from build123d import *

# Parameters (mm, degrees)
F0_W      = 13.3
F0_H      = 8.82
F1_DEPTH  = 6.28
F2_R      = 3.95
F3_DEPTH  = 13.3
F4_W      = 8.82
F4_H      = 11.06
F5_DEPTH  = 3.54
F6_R      = 0.25
F7_W      = 4.685
F7_H      = 5.95
F9_R      = 3.25
F10_DEPTH = 9.4
F11_R     = 0.75
F12_DEPTH = 7.85
F13_R     = 0.875
F14_DEPTH = 1.5


with BuildPart() as f1:
    # F0 (on Top) → F1 (new body)
    with BuildSketch(Plane.XY):
        Rectangle(F0_W, F0_H)
    extrude(amount=F1_DEPTH)

    # F2 (on face) → F3 (join, through all)
    with BuildSketch(Plane.YZ.offset(6.65)):
        with Locations((0, 6.28)):
            Circle(F2_R)
    extrude(amount=-F3_DEPTH)

    # F4 (on face) → F5 (join)
    with BuildSketch(Plane(origin=(-6.65, 0, 0), x_dir=(0, -1, 0), z_dir=(-1, 0, 0))):
        with Locations((0, 5.53)):
            Rectangle(F4_W, F4_H)
    extrude(amount=-F5_DEPTH)

    # F6
    f6_edges = [f1.edges().sort_by_distance(p)[0] for p in [
        (-6.65, 0, 11.06),
        (-6.65, 4.41, 5.53),
        (-6.65, 0, 0),
        (-6.65, -4.41, 5.53),
    ]]
    fillet(f6_edges, radius=F6_R)

    # F7 (on face) → F8 (join, up to the next surface of F1)
    with BuildSketch(Plane.XY.offset(11.06)):
        with Locations((-0.7675, 0)):
            Rectangle(F7_W, F7_H)
        with BuildLine():
            Line((1.575, 2.975), (1.575, -2.975))
            ThreePointArc((1.575, -2.975), (4.55, 0), (1.575, 2.975))
        make_face()
    extrude(until=Until.NEXT, dir=(0, 0, -1))

    # F9 (on face) → F10 (cut)
    with BuildSketch(Plane(origin=(-6.65, 0, 0), x_dir=(0, -1, 0), z_dir=(-1, 0, 0))):
        with Locations((0, 6.5)):
            Circle(F9_R)
    extrude(amount=-F10_DEPTH, mode=Mode.SUBTRACT)

    # F11 (on face) → F12 (join)
    with BuildSketch(Plane(origin=(2.75, 0, 0), x_dir=(0, -1, 0), z_dir=(-1, 0, 0))):
        with Locations((0, 6.5)):
            Circle(F11_R)
    extrude(amount=F12_DEPTH)

    # F13 (on face) → F14 (join)
    with BuildSketch(Plane(origin=(0, 0, 0), x_dir=(1, 0, 0), z_dir=(0, 0, -1))):
        with Locations((-1.425, 0)):
            Circle(F13_R)
        with Locations((3.275, 0)):
            Circle(F13_R)
    extrude(amount=F14_DEPTH)


solid = f1.part
Can you work these out from the model? Positions are in its coordinate system, mm. A direction names the side the tool comes from. Coordinates: 2 decimals unless noted, no trailing zeros. Loops run counter-clockwise (first coordinate to the right, second up) from the corner with the lowest first, then second, coordinate; pieces in that order, holes last. Notation, with made-up numbers: M 87,29 L 144,29 A19 ccw 144,38 Z; hole C -2.75,-27.75 d8. An arc over 180 degrees is marked long. Answer as CSV lines item,"result". Start each with the question number.
1. Suppose I cut it at D-D, the plane x = 4.75. List the corners of the cut face in (y, z) for me, plus the area to 3 significant figures.
2. Suppose I cut it at A-A, the plane x = -4.5. List the corners of the cut face in (y, z) for me.
3. If I drill on probe 1 along Z at (x, y) = (-2.25, 0); probe 2 along Z at (x, y) = (0.75, 0); probe 3 along Y at (x, z) = (-5.75, 7.75), over which ranges is the centre line in solid material (lowest first)? Write a range as [from, to].
4. Suppose I cut it at B-B, the plane y = 0. List the corners of the cut face in (x, z) for me.
5. For faces 1 (the face through (-1, -2.975, 10)), 2 (the face through (2.4, 0, -0.7)), 3 (the face through (-1, 2.975, 10)), 4 (the face through (-1.12, 0.163, 5.768)), which set-ups out of +Z, -Z, +X, -X, +Y, -Y let a thin tool reach every point of the face, with its end or its side?
6. Suppose I cut it at C-C, the plane z = 9.25. List the corners of the cut face in (x, y) for me (3 decimals).
7. For pin 1 Ø1.1 at (x, z) = (-1.5, 9.5) entering from +Y (3 decimals); pin 2 Ø3 at (y, z) = (0.5, 8) entering from -X; pin 3 Ø0.7 at (x, z) = (-1.5, 9.5) entering from -Y (3 decimals), each with a flat end and sliding along its axis, tell me the tip position at first contact or that it passes through.
8. Thinking about a two-plate mould opening in Z: for faces 5 (the face through (-5.1, 0, 7)), 6 (the face through (-6.65, 1, 3)), 7 (the face through (2.75, 1, 7)), 8 (the face through (3, 0, -1.5)), which applies, +Z half, -Z half, draft (parallel to the pull), parting line (faces both ways), or undercut?
Output:
1,outline,"M -4.41,0 L 4.41,0 L 4.41,6.28 L 3.95,6.28 A3.95 ccw -3.95,6.28 L -4.41,6.28 Z"
1,area,"79.9 mm^2"
2,outline,"M -4.41,0 L 4.41,0 L 4.41,11.06 L -4.41,11.06 Z; C 0,6.5 d1.5; hole C 0,6.5 d6.5"
3,probe 1,"z = [-1.5, 3.25], [5.75, 7.25], [9.75, 11.06]"
3,probe 2,"z = [0, 3.25], [5.75, 7.25], [9.75, 11.06]"
3,probe 3,"y = [-4.41, -3], [3, 4.41]"
4,outline,"M -6.65,0.25 A0.25 ccw -6.4,0 L -2.3,0 L -2.3,-1.5 L -0.55,-1.5 L -0.55,0 L 2.4,0 L 2.4,-1.5 L 4.15,-1.5 L 4.15,0 L 6.65,0 L 6.65,10.23 L 4.55,10.23 L 4.55,11.06 L -6.4,11.06 A0.25 ccw -6.65,10.81 L -6.65,9.75 L 2.75,9.75 L 2.75,7.25 L -5.1,7.25 L -5.1,5.75 L 2.75,5.75 L 2.75,3.25 L -6.65,3.25 Z"
5,face 1,"+Z, +X, -Y"
5,face 2,"-Z"
5,face 3,"+Z, +X, +Y"
5,face 4,"-X"
6,outline,"M -6.65,-4.16 A0.25 ccw -6.4,-4.41 L -3.11,-4.41 L -3.11,-2.975 L 1.575,-2.975 A2.975 ccw 3.013,-2.604 L 6.65,-2.604 L 6.65,2.604 L 3.013,2.604 A2.975 ccw 1.575,2.975 L -3.11,2.975 L -3.11,4.41 L -6.4,4.41 A0.25 ccw -6.65,4.16 L -6.65,1.732 L 2.75,1.732 L 2.75,-1.732 L -6.65,-1.732 Z"
7,pin 1,"stops at y = 2.975"
7,pin 2,"stops at x = -5.1"
7,pin 3,"stops at y = -2.975"
8,face 5,"undercut"
8,face 6,"draft"
8,face 7,"undercut"
8,face 8,"-Z half"
